The model under review builds one solid part; all positions refer to its coordinate system, in mm. A direction names the side the tool comes from. Coordinates: 2 decimals unless noted, no trailing zeros. Order: outer loops, then holes, each group sorted by start corner. A loop starts at its lowest first (then second) coordinate and runs counter-clockwise, first axis right, second up. Notation, with made-up numbers: (59, 50.5) - (70, 50.5) arc R23 cw to (70, 69.5) - close; hole circle Ø7 at (83, 38). An arc over 180 degrees is marked (long way). Answer in a Markdown table with one row per item.
Autodesk Fusion 360 part; units mm, degrees
sketch "Sketch1" plane through (0, 0, 0) normal (0, 0, 1) x (1, 0, 0)
  line L0 (0, 0) -> (0, 260)
  line L1 (0, 0) -> (-30, 0)
  line L2 (-30, 0) -> (0, 0)
  line L3 (0, 0) -> (0, 10)
  line L4 (0, 10) -> (-30, 10)
  line L5 (-30, 10) -> (-30, 0)
  line L6 (0, 10) -> (-10, 10)
  line L7 (-10, 10) -> (-10, 280)
  line L8 (-10, 280) -> (40, 280)
  line L9 (40, 280) -> (40, 260)
  line L10 (40, 260) -> (-10, 260)
  line L11 (-10, 260) -> (-10, 280)
  dimension "d1" = 260
  dimension "d2" = 30
  dimension "d3" = 10
  dimension "d4" = 270
  dimension "d5" = 50
  dimension "d6" = 20
extrude "Extrude1" add sketch "Sketch1" along normal blind 20
sketch "Sketch2" plane through (0, 260, 0) normal (0, -1, 0) x (1, 0, 0)
  line L0 (0, 0) -> (40, 0)
  line L1 (40, 0) -> (40, 20)
  line L2 (40, 20) -> (0, 20)
  line L3 (0, 20) -> (0, 0)
  line L4 (20, 20) -> (20, 10)
  circle A0 centre (20, 10) radius 5
  dimension "d9" = 10
sketch "Sketch3" plane through (0, 10, 0) normal (0, 1, 0) x (-1, 0, 0)
  line L0 (10, 0) -> (30, 0)
  line L1 (30, 0) -> (30, 20)
  line L2 (30, 20) -> (10, 20)
  line L3 (10, 20) -> (10, 0)
  circle A0 centre (20, 10) radius 5
  dimension "d10" = 10
extrude "Extrude2" cut sketch "Sketch3" against normal blind 25 contours A0
extrude "Extrude3" cut sketch "Sketch2" against normal blind 100 contours A0
Item 1: Clearance check with flat-ended pins moving along their axes: pin 1 Ø4 at (y, z) = (228, 4) entering from +X; pin 2 Ø10 at (y, z) = (101.5, 12) entering from -X; pin 3 Ø3 at (x, z) = (-14, 7) entering from +Y. State where each tip first meets the part, or that it passes through.
Check values:
| item | result |
|---|---|
| pin 1 | x = 0 |
| pin 2 | x = -10 |
| pin 3 | y = 10 |
Item 2: We need section A-A, the plane z = 10. Write out the cut boundary in (x, y), then the cut area to 3 significant figures.
Check values:
| item | result |
|---|---|
| outline | (-30, 0) - (-25, 0) - (-25, 10) - (-30, 10) - close; (-15, 0) - (0, 0) - (0, 260) - (15, 260) - (15, 280) - (-10, 280) - (-10, 10) - (-15, 10) - close; (25, 260) - (40, 260) - (40, 280) - (25, 280) - close |
| area | 3,500 mm^2 |
Item 3: We need section D-D, the plane y = 122.5. Write out the cut boundary in (x, z), then the cut area to 3 significant figures.
Check values:
| item | result |
|---|---|
| outline | (-10, 0) - (0, 0) - (0, 20) - (-10, 20) - close |
| area | 200 mm^2 |
Item 4: To check wall thickness, follow line 1 (X direction, y = 264.5, z = 10); line 2 (Z direction, x = 20, y = 274.75); line 3 (Y direction, x = -11, z = 10.5). State the ranges of each line that lie inside material, in increasing order. Write a range as from..to.
Check values:
| item | result |
|---|---|
| line 1 | -10..15, 25..40 |
| line 2 | 0..5, 15..20 |
| line 3 | 0..10 |
Item 5: We need section C-C, the plane x = -20. Write out the cut boundary in (y, z), then the cut area to 3 significant figures.
Check values:
| item | result |
|---|---|
| outline | (0, 0) - (10, 0) - (10, 5) - (0, 5) - close; (0, 15) - (10, 15) - (10, 20) - (0, 20) - close |
| area | 100 mm^2 |
Item 6: Tool access review of faces 1 (the face through (-10, 143, 10)), 2 (the face through (0, 128, 10)), 3 (the face through (-30, 5, 10)): name each direction out of +Z, -Z, +X, -X, +Y, -Y from which nothing blocks a thin tool from reaching the whole face with its end or side.
Check values:
| item | result |
|---|---|
| face 1 | +Z, -Z, -X, +Y |
| face 2 | +Z, -Z, +X, -Y |
| face 3 | +Z, -Z, -X, +Y, -Y |
Item 7: Mouldability with a two-part tool opening along X and no side actions: class faces 4 (the face through (-0.3, 161.4, 20)), 5 (the face through (40, 270, 10)), 6 (the face through (19.349, 269.86, 14.957)) as +X half, -X half, draft (parallel to the pull), parting line (faces both ways), or undercut.
Check values:
| item | result |
|---|---|
| face 4 | draft |
| face 5 | +X half |
| face 6 | undercut |
Item 8: We need section B-B, the plane x = 20. Write out the cut boundary in (y, z), then the cut area to 3 significant figures.
Check values:
| item | result |
|---|---|
| outline | (260, 0) - (280, 0) - (280, 5) - (260, 5) - close; (260, 15) - (280, 15) - (280, 20) - (260, 20) - close |
| area | 200 mm^2 |
